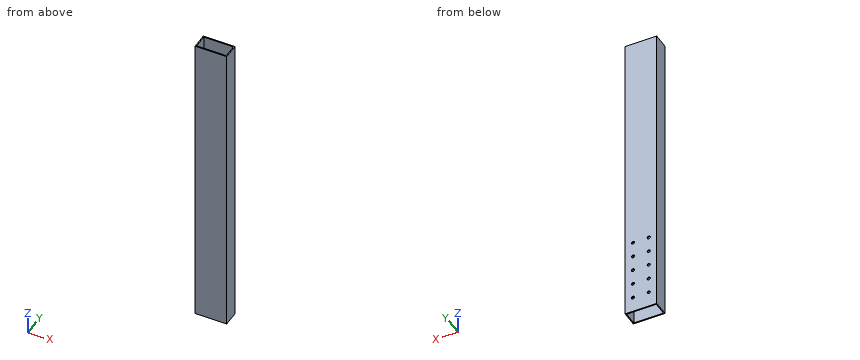
```python
from build123d import *

# Parameters (mm, degrees)
SKETCH1_W           = 50.8
SKETCH1_H           = 25.4
BOSS_EXTRUDE1_DEPTH = 495.3
SHELL1_T            = -1.5875
CUT_EXTRUDE1_REACH  = 498.601
SKETCH2_R           = 2.4892


with BuildPart() as part:
    # Sketch1 → Boss-Extrude1 (new body)
    with BuildSketch(Plane.XY):
        Rectangle(SKETCH1_W, SKETCH1_H)
    extrude(amount=BOSS_EXTRUDE1_DEPTH)

    # Shell1
    shell1_openings = [part.faces().sort_by_distance(p)[0] for p in [
        (0, 0, 495.3),
        (0, 0, 0),
    ]]
    offset(amount=SHELL1_T, openings=shell1_openings, kind=Kind.INTERSECTION)

    # Sketch2 → Cut-Extrude1 (cut, up to next)
    with BuildSketch(Plane(origin=(0, 12.7, 0), x_dir=(1, 0, 0), z_dir=(0, 1, 0)), mode=Mode.PRIVATE) as cut_extrude1_sk1:
        with Locations(Location((-12.7, -25.4, 0), (0, 0, 270))):
            Circle(SKETCH2_R)
    cut_extrude1_tool1 = extrude(cut_extrude1_sk1.sketch, amount=-CUT_EXTRUDE1_REACH, mode=Mode.PRIVATE) & part.part
    # Sketch2 → Cut-Extrude1 (cut, up to next)
    with BuildSketch(Plane(origin=(0, 12.7, 0), x_dir=(1, 0, 0), z_dir=(0, 1, 0)), mode=Mode.PRIVATE) as cut_extrude1_sk2:
        with Locations(Location((12.7, -25.4, 0), (0, 0, 270))):
            Circle(SKETCH2_R)
    cut_extrude1_tool2 = extrude(cut_extrude1_sk2.sketch, amount=-CUT_EXTRUDE1_REACH, mode=Mode.PRIVATE) & part.part
    # Sketch2 → Cut-Extrude1 (cut, up to next)
    with BuildSketch(Plane(origin=(0, 12.7, 0), x_dir=(1, 0, 0), z_dir=(0, 1, 0)), mode=Mode.PRIVATE) as cut_extrude1_sk3:
        with Locations(Location((12.7, -50.8, 0), (0, 0, 270))):
            Circle(SKETCH2_R)
    cut_extrude1_tool3 = extrude(cut_extrude1_sk3.sketch, amount=-CUT_EXTRUDE1_REACH, mode=Mode.PRIVATE) & part.part
    # Sketch2 → Cut-Extrude1 (cut, up to next)
    with BuildSketch(Plane(origin=(0, 12.7, 0), x_dir=(1, 0, 0), z_dir=(0, 1, 0)), mode=Mode.PRIVATE) as cut_extrude1_sk4:
        with Locations(Location((12.7, -76.2, 0), (0, 0, 270))):
            Circle(SKETCH2_R)
    cut_extrude1_tool4 = extrude(cut_extrude1_sk4.sketch, amount=-CUT_EXTRUDE1_REACH, mode=Mode.PRIVATE) & part.part
    # Sketch2 → Cut-Extrude1 (cut, up to next)
    with BuildSketch(Plane(origin=(0, 12.7, 0), x_dir=(1, 0, 0), z_dir=(0, 1, 0)), mode=Mode.PRIVATE) as cut_extrude1_sk5:
        with Locations(Location((12.7, -101.6, 0), (0, 0, 270))):
            Circle(SKETCH2_R)
    cut_extrude1_tool5 = extrude(cut_extrude1_sk5.sketch, amount=-CUT_EXTRUDE1_REACH, mode=Mode.PRIVATE) & part.part
    # Sketch2 → Cut-Extrude1 (cut, up to next)
    with BuildSketch(Plane(origin=(0, 12.7, 0), x_dir=(1, 0, 0), z_dir=(0, 1, 0)), mode=Mode.PRIVATE) as cut_extrude1_sk6:
        with Locations(Location((12.7, -127, 0), (0, 0, 270))):
            Circle(SKETCH2_R)
    cut_extrude1_tool6 = extrude(cut_extrude1_sk6.sketch, amount=-CUT_EXTRUDE1_REACH, mode=Mode.PRIVATE) & part.part
    # Sketch2 → Cut-Extrude1 (cut, up to next)
    with BuildSketch(Plane(origin=(0, 12.7, 0), x_dir=(1, 0, 0), z_dir=(0, 1, 0)), mode=Mode.PRIVATE) as cut_extrude1_sk7:
        with Locations(Location((-12.7, -50.8, 0), (0, 0, 270))):
            Circle(SKETCH2_R)
    cut_extrude1_tool7 = extrude(cut_extrude1_sk7.sketch, amount=-CUT_EXTRUDE1_REACH, mode=Mode.PRIVATE) & part.part
    # Sketch2 → Cut-Extrude1 (cut, up to next)
    with BuildSketch(Plane(origin=(0, 12.7, 0), x_dir=(1, 0, 0), z_dir=(0, 1, 0)), mode=Mode.PRIVATE) as cut_extrude1_sk8:
        with Locations(Location((-12.7, -76.2, 0), (0, 0, 270))):
            Circle(SKETCH2_R)
    cut_extrude1_tool8 = extrude(cut_extrude1_sk8.sketch, amount=-CUT_EXTRUDE1_REACH, mode=Mode.PRIVATE) & part.part
    # Sketch2 → Cut-Extrude1 (cut, up to next)
    with BuildSketch(Plane(origin=(0, 12.7, 0), x_dir=(1, 0, 0), z_dir=(0, 1, 0)), mode=Mode.PRIVATE) as cut_extrude1_sk9:
        with Locations(Location((-12.7, -101.6, 0), (0, 0, 270))):
            Circle(SKETCH2_R)
    cut_extrude1_tool9 = extrude(cut_extrude1_sk9.sketch, amount=-CUT_EXTRUDE1_REACH, mode=Mode.PRIVATE) & part.part
    # Sketch2 → Cut-Extrude1 (cut, up to next)
    with BuildSketch(Plane(origin=(0, 12.7, 0), x_dir=(1, 0, 0), z_dir=(0, 1, 0)), mode=Mode.PRIVATE) as cut_extrude1_sk10:
        with Locations(Location((-12.7, -127, 0), (0, 0, 270))):
            Circle(SKETCH2_R)
    cut_extrude1_tool10 = extrude(cut_extrude1_sk10.sketch, amount=-CUT_EXTRUDE1_REACH, mode=Mode.PRIVATE) & part.part
    add(cut_extrude1_tool1.solids().sort_by_distance((-12.7, 12.7, 25.4))[0], mode=Mode.SUBTRACT)
    add(cut_extrude1_tool2.solids().sort_by_distance((12.7, 12.7, 25.4))[0], mode=Mode.SUBTRACT)
    add(cut_extrude1_tool3.solids().sort_by_distance((12.7, 12.7, 50.8))[0], mode=Mode.SUBTRACT)
    add(cut_extrude1_tool4.solids().sort_by_distance((12.7, 12.7, 76.2))[0], mode=Mode.SUBTRACT)
    add(cut_extrude1_tool5.solids().sort_by_distance((12.7, 12.7, 101.6))[0], mode=Mode.SUBTRACT)
    add(cut_extrude1_tool6.solids().sort_by_distance((12.7, 12.7, 127))[0], mode=Mode.SUBTRACT)
    add(cut_extrude1_tool7.solids().sort_by_distance((-12.7, 12.7, 50.8))[0], mode=Mode.SUBTRACT)
    add(cut_extrude1_tool8.solids().sort_by_distance((-12.7, 12.7, 76.2))[0], mode=Mode.SUBTRACT)
    add(cut_extrude1_tool9.solids().sort_by_distance((-12.7, 12.7, 101.6))[0], mode=Mode.SUBTRACT)
    add(cut_extrude1_tool10.solids().sort_by_distance((-12.7, 12.7, 127))[0], mode=Mode.SUBTRACT)


solid = part.part
```
Read the model definition and answer for the solid it produces. Units are mm, in the model's axes. Give positions to 0.01 mm unless a question says otherwise; leave off trailing zeros. Loops run counter-clockwise (first coordinate to the right, second up) from the corner with the lowest first, then second, coordinate; pieces in that order, holes last.
Item 1: The part is cut by section A-A (z = 151). Write down the section's boundary in (x, y).
Item 2: Each of these flat-tipped pins is pushed along its axis until it touches: pin 1 Ø3 at (x, z) = (-12.7, 25.4) entering from +Y; pin 2 Ø6 at (x, y) = (20, 2) entering from +Z; pin 3 Ø8 at (x, z) = (12.7, 50.8) entering from +Y. Where does it stop, or does it pass through?
Item 3: The part is cut by section B-B (y = 3.5). Write down the section's boundary in (x, z).
Item 4: Find the intervals of material crossed by line 1 along X through (y, z) = (11.65, 127); line 2 along Y through (x, z) = (3, 202); line 3 along X through (y, z) = (3.25, 266), in increasing order.
Taken from the geometry:
1. outline: (-25.4, -12.7) - (25.4, -12.7) - (25.4, 12.7) - (-25.4, 12.7) - close; hole (-23.81, -11.11) - (23.81, -11.11) - (23.81, 11.11) - (-23.81, 11.11) - close
2. pin 1: stops at y = -11.11
2. pin 2: passes through
2. pin 3: stops at y = 12.7
3. outline: (-25.4, 0) - (-23.81, 0) - (-23.81, 495.3) - (-25.4, 495.3) - close; (23.81, 0) - (25.4, 0) - (25.4, 495.3) - (23.81, 495.3) - close
4. line 1: x = -25.4 to -15.19, -10.21 to 10.21, 15.19 to 25.4
4. line 2: y = -12.7 to -11.11, 11.11 to 12.7
4. line 3: x = -25.4 to -23.81, 23.81 to 25.4
